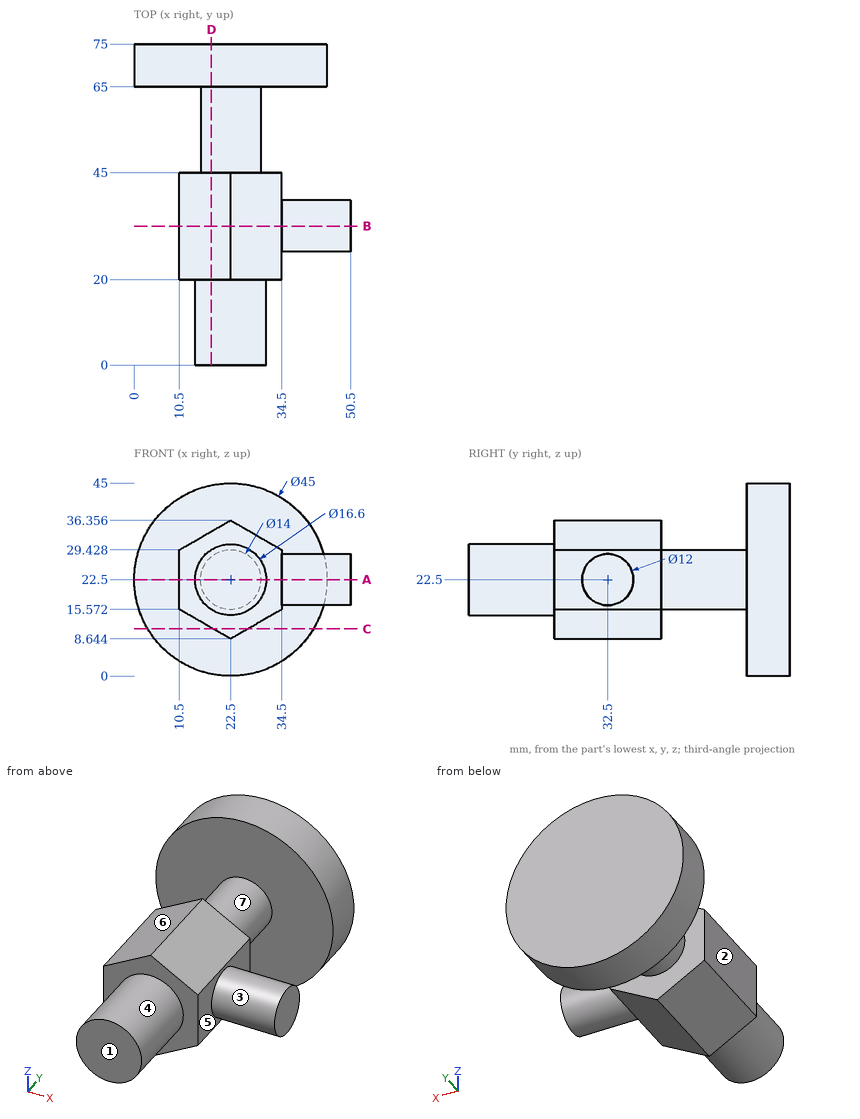
Design review of the part shown in the three views and the two pictorial views. Dimensions are in mm from the part's minimum x, y and z. A direction names the side the tool comes from. Round coordinates to 2 decimals unless told otherwise and drop trailing zeros. Write each loop counter-clockwise with the first axis right and the second up, starting at its lowest first coordinate (ties: lowest second). Pieces come first, ordered by that corner, then holes. Notation, with made-up numbers: (4, 81.25) -> (62, 81.25) arc R11 ccw to (62, 92.25) -> close; hole circle Ø5 at (27, 78.25). An arc over 180 degrees is marked (long way). Write item = value, one per line. Start each with the question number.
1) Take a section at A-A, the plane z = 22.5. State the section outline as (x, y) points.
2) Clearance check with flat-ended pins moving along their axes: pin 1 (3 mm diameter, centred on y = 24, z = 10.5, fed in from -X) (1 decimal); pin 2 (2 mm diameter, centred on x = 44, y = 32, fed in from -Z); pin 3 (1.5 mm diameter, centred on x = 15.5, z = 29.5, fed in from -Y). State where each tip first meets the part, or that it passes through.
3) Tool access review of the marked faces 4, 5, 6 and 7: name each direction out of +Z, -Z, +X, -X, +Y, -Y from which nothing blocks a thin tool from reaching the whole face with its end or side.
4) Take a section at D-D, the plane x = 18. State the section outline as (y, z) points (1 decimal).
5) Mouldability with a two-part tool opening along Y and no side actions: class the marked faces 1, 2 and 3 as +Y half, -Y half, draft (parallel to the pull), parting line (faces both ways), or undercut.
6) Take a section at B-B, the plane y = 32.5. State the section outline as (x, z) points.
7) Take a section at C-C, the plane z = 11. State the section outline as (x, y) points.
8) Wall thickness on probe 1 along Y at (x, z) = (28, 31); probe 2 along Y at (x, z) = (27.5, 16.5); probe 3 along Y at (x, z) = (20, 2.5): over which ranges is each line inside the solid? List them lowest first. Write a range as from..to.
Results list:
q1.outline = (0, 65) -> (15.5, 65) -> (15.5, 45) -> (10.5, 45) -> (10.5, 20) -> (14.2, 20) -> (14.2, 0) -> (30.8, 0) -> (30.8, 20) -> (34.5, 20) -> (34.5, 26.5) -> (50.5, 26.5) -> (50.5, 38.5) -> (34.5, 38.5) -> (34.5, 45) -> (29.5, 45) -> (29.5, 65) -> (45, 65) -> (45, 75) -> (0, 75) -> close
q2.pin_1 = 16.7
q2.pin_2 = 16.5
q2.pin_3 = 20
q3.face_4 = -Y
q3.face_5 = +X
q3.face_6 = +Z, -X, -Y
q3.face_7 = none
q4.outline = (0, 15.5) -> (20, 15.5) -> (20, 11.2) -> (45, 11.2) -> (45, 17.1) -> (65, 17.1) -> (65, 0.5) -> (75, 0.5) -> (75, 44.5) -> (65, 44.5) -> (65, 27.9) -> (45, 27.9) -> (45, 33.8) -> (20, 33.8) -> (20, 29.5) -> (0, 29.5) -> close
q5.face_1 = -Y half
q5.face_2 = draft
q5.face_3 = undercut
q6.outline = (10.5, 15.57) -> (22.5, 8.64) -> (34.5, 15.57) -> (34.5, 16.5) -> (50.5, 16.5) -> (50.5, 28.5) -> (34.5, 28.5) -> (34.5, 29.43) -> (22.5, 36.36) -> (10.5, 29.43) -> close
q7.outline = (3.16, 65) -> (41.84, 65) -> (41.84, 75) -> (3.16, 75) -> close; (18.42, 20) -> (26.58, 20) -> (26.58, 45) -> (18.42, 45) -> close
q8.probe_1 = 20..45, 65..75
q8.probe_2 = 0..45, 65..75
q8.probe_3 = 65..75
